Print and shaded views of the part. All mm, measured from the part's lowest x, y and z. A direction names the side the tool comes from. Coordinates: 2 decimals unless noted, no trailing zeros. Loops run counter-clockwise (first coordinate to the right, second up) from the corner with the lowest first, then second, coordinate; pieces in that order, holes last. Notation, with made-up numbers: M 31.5,28 L 37.5,28 A17 cw 37.5,61 Z; hole C -4,37.25 d5. An arc over 180 degrees is marked long. One line per question, with ' | ' between items. Start each with the question number.
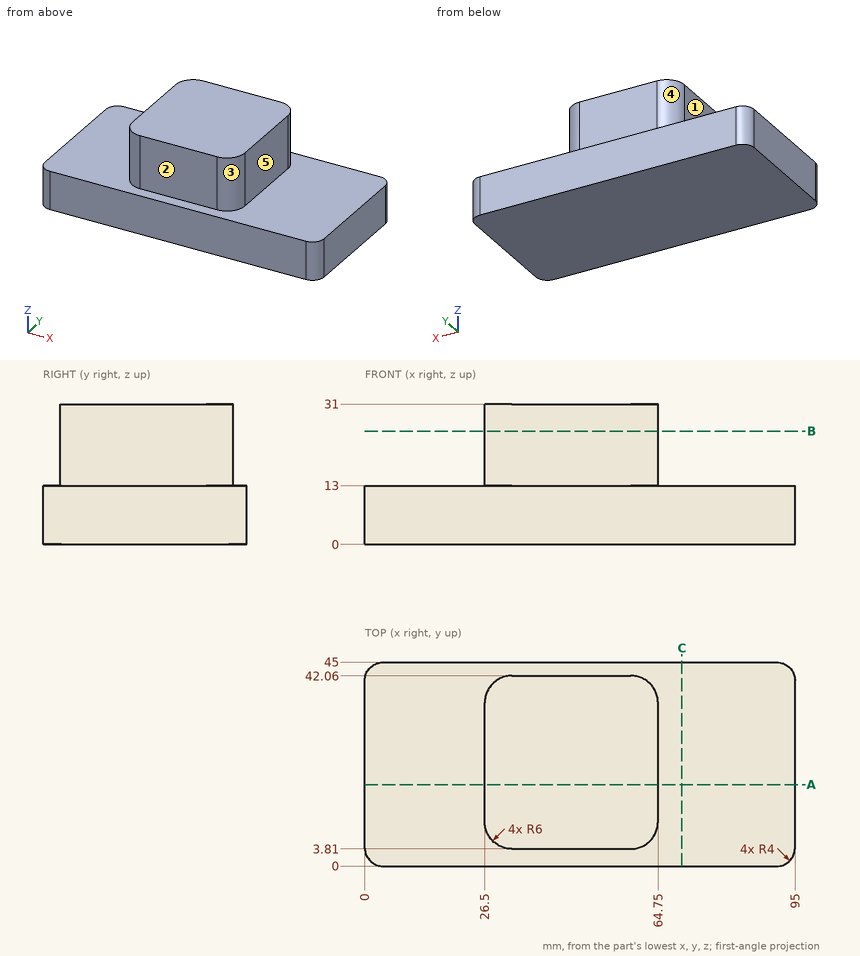
(1) Band-saw the part on B-B on z = 25. Write the cut outline in (x, y), then the cut area to 3 significant figures.
(2) 3-axis set-ups, long thin cutter, end or side, ignore diameter. For the marked faces 1, 2, 3, 4 and 5: which of +Z, -Z, +X, -X, +Y, -Y reach the whole face in a straight line?
(3) Pin check, flat tips, straight feed: P1, Ø1.5, axis at x = 9.5, y = 25.5, coming from the +Z side; P2, Ø8, axis at y = 24.5, z = 22, coming from the -X side; P3, Ø1.5, axis at x = 45, z = 26, coming from the -Y side. Stop position of each tip, or through.
(4) Band-saw the part on C-C on x = 70. Write the cut outline in (y, z).
(5) Band-saw the part on A-A on y = 18. Write the cut outline in (x, z).
(6) Drill centre lines: line 1 (X direction, y = 13.5, z = 28); line 2 (Y direction, x = 43, z = 18.5); line 3 (Z direction, x = 59, y = 3). Where is each one in solid material? Low to high. Write a range as [from, to].
Computed values:
1) outline: M 26.5,9.81 A6 ccw 32.5,3.81 L 58.75,3.81 A6 ccw 64.75,9.81 L 64.75,36.06 A6 ccw 58.75,42.06 L 32.5,42.06 A6 ccw 26.5,36.06 Z | area: 1,430 mm^2
2) face 1: +Z, -X, +Y, -Y | face 2: +Z, +X, -X, -Y | face 3: +Z, +X, -Y | face 4: +Z, -X, +Y | face 5: +Z, +X, +Y, -Y
3) P1: z = 13 | P2: x = 26.5 | P3: y = 3.81
4) outline: M 0,0 L 45,0 L 45,13 L 0,13 Z
5) outline: M 0,0 L 95,0 L 95,13 L 64.75,13 L 64.75,31 L 26.5,31 L 26.5,13 L 0,13 Z
6) line 1: [26.5, 64.75] | line 2: [3.81, 42.06] | line 3: [0, 13]
